Design review of the part built by this model. Coordinates are the model's own, in mm. A direction names the side the tool comes from. Round coordinates to 2 decimals unless told otherwise and drop trailing zeros. Loops run counter-clockwise (first coordinate to the right, second up) from the corner with the lowest first, then second, coordinate; pieces in that order, holes last. Notation, with made-up numbers: M 57,50.5 L 81,50.5 A18 ccw 81,79.5 Z; hole C 19.5,40.25 d10. An arc over 180 degrees is marked long. One line per item, written item: value. Start each with the question number.
Item 1: For line 1 along Y through (x, z) = (-13, -50); line 2 along X through (y, z) = (-44, 2); line 3 along X through (y, z) = (8.5, 7.5), list the stretches that pass through material, from the lowest coordinate up.
Item 2: We need section A-A (x = 30). Write out the cut boundary in (y, z), then the cut area to 3 significant figures.
Item 3: Mouldability with a two-part tool opening along X and no side actions: class faces 6 (the flat face through (-34, -39, 5)), 7 (the cylindrical face through (-15.542, -26.976, -49.909)), 8 (the cylindrical face through (-49, -26, -13)) as released by +X, released by -X, zero draft, split by the parting line, or undercut.
Item 4: We need section C-C (y = -44.5). Write out the cut boundary in (x, z).
Item 5: We need section D-D (z = -50.15). Write out the cut boundary in (x, y).
Item 6: Clearance check with flat-ended pins moving along their axes: pin 1 (12 mm diameter, centred on x = -17, z = -27, fed in from +Y); pin 2 (10 mm diameter, centred on x = 13, y = -21.5, fed in from -Z); pin 3 (2.5 mm diameter, centred on x = 29, y = -1, fed in from +Z). State where each tip first meets the part, or that it passes through.
Item 7: For faces 1 (the flat face through (-42.5, -33, 5)), 2 (the flat face through (-43, 4, 0)), 3 (the flat face through (-9, 7.84, -28)), 4 (the flat face through (-18.5, -20.13, -44.35)), 5 (the flat face through (-16, -36, -51.3)), list the 3-axis set-ups (+Z, -Z, +X, -X, +Y, -Y) from which the entire face can be reached by the end or side of a thin tool; tool diameter is ignored.
from build123d import *

# Parameters (mm, degrees)
SKETCH1_W            = 100
SKETCH1_H            = 60
SKETCH1_R            = 4.25
BOSS_EXTRUDE1_DEPTH  = 13.5
SKETCH2_R            = 7
BOSS_EXTRUDE2_DEPTH  = 10
CHAMFER1_SIZE        = 14
FILLET1_R            = 2.5
CUT_EXTRUDE1_DEPTH   = 12
SKETCH5_R            = 1.25
CUT_EXTRUDE2_DEPTH   = 12
SKETCH6_R            = 2.75
CUT_EXTRUDE3_DEPTH   = 10
CUT_EXTRUDE4_DEPTH   = 17
SKETCH11_W           = 17
SKETCH11_H           = 28.01
CUT_EXTRUDE5_DEPTH   = 28.0000001
SKETCH13_R           = 4.25
BOSS_EXTRUDE6_DEPTH  = 9
SKETCH14_R           = 1.85
SKETCH14_R_2         = 11.7
BOSS_EXTRUDE7_DEPTH  = 6
BOSS_EXTRUDE8_START  = 4
BOSS_EXTRUDE8_DEPTH  = 3
SKETCH17_W           = 6
SKETCH17_H           = 42.718705864
BOSS_EXTRUDE9_DEPTH  = 1
BOSS_EXTRUDE12_DEPTH = 3
SKETCH19_W           = 6
SKETCH19_H           = 24.5
BOSS_EXTRUDE13_DEPTH = 6
SKETCH21_W           = 6
SKETCH21_H           = 21.281155669
BOSS_EXTRUDE14_DEPTH = 3
BOSS_EXTRUDE15_DEPTH = 3
FILLET3_R            = 2


with BuildPart() as part:
    # Sketch1 → Boss-Extrude1 (new body, symmetric)
    with BuildSketch(Plane.XY):
        with Locations((0, -19)):
            Rectangle(SKETCH1_W, SKETCH1_H)
        with Locations((30, 0)):
            Circle(SKETCH1_R, mode=Mode.SUBTRACT)
        with Locations((-30, 0)):
            Circle(SKETCH1_R, mode=Mode.SUBTRACT)
    extrude(amount=BOSS_EXTRUDE1_DEPTH, both=True)

    # Sketch2 → Boss-Extrude2 (add)
    with BuildSketch(Plane(origin=(0, 0, -13.5), x_dir=(-1, 0, 0), z_dir=(0, 0, -1))):
        with Locations((-30, 0)):
            Circle(SKETCH2_R)
        with Locations((30, 0)):
            Circle(SKETCH2_R)
    extrude(amount=-BOSS_EXTRUDE2_DEPTH)

    # Chamfer1
    chamfer1_edges = [part.edges().sort_by_distance(p)[0] for p in [
        (-50, 11, 0),
        (50, 11, 0),
    ]]
    chamfer(chamfer1_edges, length=CHAMFER1_SIZE)

    # Fillet1
    fillet1_edges = [part.edges().sort_by_distance(p)[0] for p in [
        (-50, -26, -13.5),
        (-50, -26, 13.5),
        (0, 11, -13.5),
        (43, 4, -13.5),
        (-43, 4, -13.5),
        (0, 11, 13.5),
        (50, -26, 13.5),
        (43, 4, 13.5),
        (-43, 4, 13.5),
        (50, -26, -13.5),
    ]]
    fillet(fillet1_edges, radius=FILLET1_R)

    # Sketch3 → Cut-Extrude1 (cut)
    with BuildSketch(Plane.XY.offset(13.5)):
        Polygon((11.5, 1.5), (-11.5, 1.5), (-11.5, -14.75), (-11.5, -25.79), (11.5, -25.79), (11.5, -14.75), align=None)
    extrude(amount=-CUT_EXTRUDE1_DEPTH, mode=Mode.SUBTRACT)

    # Sketch5 → Cut-Extrude2 (cut)
    with BuildSketch(Plane(origin=(0, 11, 0), x_dir=(1, 0, 0), z_dir=(0, 1, 0))):
        with Locations((30, -7.5)):
            Circle(SKETCH5_R)
        with Locations((-30, -7.5)):
            Circle(SKETCH5_R)
    extrude(amount=-CUT_EXTRUDE2_DEPTH, mode=Mode.SUBTRACT)

    # Sketch6 → Cut-Extrude3 (cut)
    with BuildSketch(Plane.XZ.offset(49)):
        with Locations((36.277796695, 2.75)):
            Circle(SKETCH6_R)
    cut_extrude3 = extrude(amount=-CUT_EXTRUDE3_DEPTH, mode=Mode.SUBTRACT)

    # Sketch7 → Cut-Extrude4 (cut)
    with BuildSketch(Plane.XY.offset(13.5)):
        Polygon((42.5, -39), (30.5, -39), (25.5, -39), (25.5, -28), (30.5, -28), (42.5, -28), align=None)
    cut_extrude4 = extrude(amount=-CUT_EXTRUDE4_DEPTH, mode=Mode.SUBTRACT)

    # Mirror1: Cut-Extrude3, Cut-Extrude4 across plane
    add(cut_extrude3.mirror(Plane(origin=(0, 0, 0), x_dir=(0, 0, 1), z_dir=(1, 0, 0))), mode=Mode.SUBTRACT)
    add(cut_extrude4.mirror(Plane(origin=(0, 0, 0), x_dir=(0, 0, 1), z_dir=(1, 0, 0))), mode=Mode.SUBTRACT)

    # Sketch11 → Cut-Extrude5 (cut, through all)
    with BuildSketch(Plane(origin=(0, 0, -13.5), x_dir=(-1, 0, 0), z_dir=(0, 0, -1))):
        with Locations((0, -13.310174912)):
            Rectangle(SKETCH11_W, SKETCH11_H)
    extrude(amount=-CUT_EXTRUDE5_DEPTH, mode=Mode.SUBTRACT)

    # Sketch13 → Boss-Extrude6 (add)
    with BuildSketch(Plane.XY.offset(-3.5)):
        with Locations((30, 0)):
            Circle(SKETCH13_R)
        with Locations((-30, 0)):
            Circle(SKETCH13_R)
    extrude(amount=BOSS_EXTRUDE6_DEPTH)

    # Sketch14 → Boss-Extrude7 (add)
    with BuildSketch(Plane(origin=(-18.5, 0, 0), x_dir=(0, 0, -1), z_dir=(1, 0, 0))):
        Polygon((55.8, -29.960174912), (55.8, 3.339825088), (51.3, 7.839825088), (18, 7.839825088), (11, 7.839825088), (11, -34.460174912), (18, -34.460174912), (51.3, -34.460174912), align=None)
        with Locations((50.15, -28.810174912)):
            Circle(SKETCH14_R, mode=Mode.SUBTRACT)
        with Locations((50.15, 2.189825088)):
            Circle(SKETCH14_R, mode=Mode.SUBTRACT)
        with Locations((19.15, 2.189825088)):
            Circle(SKETCH14_R, mode=Mode.SUBTRACT)
        with Locations((19.15, -28.810174912)):
            Circle(SKETCH14_R, mode=Mode.SUBTRACT)
        with Locations((34.65, -13.310174912)):
            Circle(SKETCH14_R_2, mode=Mode.SUBTRACT)
    extrude(amount=BOSS_EXTRUDE7_DEPTH)

    # Sketch15 → Boss-Extrude8 (add)
    with BuildSketch(Plane.XZ.offset(34.460174912).offset(BOSS_EXTRUDE8_START)):
        Polygon((-14.5, -39.5), (20.060854185, -10.5), (-14.5, -10.5), align=None)
    extrude(amount=-BOSS_EXTRUDE8_DEPTH)

    # Sketch17 → Boss-Extrude9 (add)
    with BuildSketch(Plane.XZ.offset(34.460174912)):
        with Locations((-15.5, -29.940647068)):
            Rectangle(SKETCH17_W, SKETCH17_H)
    extrude(amount=BOSS_EXTRUDE9_DEPTH)

    # Sketch18 → Boss-Extrude12 (add)
    with BuildSketch(Plane.XZ.offset(35.460174912)):
        Polygon((-18.5, -10.5), (-41.575239857, -10.5), (-18.5, -38), (-13.739171521, -38), (-13.739171521, -10.5), align=None)
    extrude(amount=BOSS_EXTRUDE12_DEPTH)

    # Sketch19 → Boss-Extrude13 (add)
    with BuildSketch(Plane.XZ.offset(38.460174912)):
        with Locations((-15.5, -25.75)):
            Rectangle(SKETCH19_W, SKETCH19_H)
    extrude(amount=-BOSS_EXTRUDE13_DEPTH)

    # Sketch21 → Boss-Extrude14 (add)
    with BuildSketch(Plane.XZ.offset(35.460174912)):
        with Locations((-15.5, -40.659422166)):
            Rectangle(SKETCH21_W, SKETCH21_H)
    extrude(amount=BOSS_EXTRUDE14_DEPTH)

    # Sketch22 → Boss-Extrude15 (add)
    with BuildSketch(Plane(origin=(0, 7.839825088, 0), x_dir=(1, 0, 0), z_dir=(0, 1, 0))):
        Polygon((-12.5, 37.821800738), (-15.5, 37.821800738), (-15.5, 11), (-12.5, 11), (16.485593407, 11), (16.485593407, 13.5), align=None)
    extrude(amount=-BOSS_EXTRUDE15_DEPTH)

    # Fillet3
    fillet3_edges = [part.edges().sort_by_distance(p)[0] for p in [
        (-12.5, 6.339825088, -37.821800738),
        (-39.057940964, -36.960174912, -13.5),
        (-18.5, -36.960174912, -38),
        (16.485593407, 6.339825088, -13.5),
        (16.485593407, -36.960174912, -13.5),
        (-12.5, -36.960174912, -37.821800738),
        (-11.286173778, -38.460174912, -13.5),
        (-12.5, -35.460174912, -25.660900369),
        (1.992796704, -35.460174912, -13.5),
        (-12.5, -15.310174912, -13.5),
        (1.992796704, 4.839825088, -13.5),
    ]]
    fillet(fillet3_edges, radius=FILLET3_R)


solid = part.part
A:
1. line 1: -38.46 to -30.65, -26.97 to 0.35, 4.03 to 7.84
1. line 2: -50 to -38.92, -33.63 to 33.63, 38.92 to 50
1. line 3: -38.5 to -31.25, -28.75 to 28.75, 31.25 to 38.5
2. outline: M -49,-13.5 L 8.5,-13.5 A2.5 ccw 11,-11 L 11,6.25 L 4.25,6.25 L 4.25,5.5 L -4.25,5.5 L -4.25,13.5 L -28,13.5 L -28,-3.5 L -39,-3.5 L -39,13.5 L -49,13.5 Z; M 4.25,8.75 L 11,8.75 L 11,11 A2.5 ccw 8.5,13.5 L 4.25,13.5 Z
2. area: 1,350 mm2
3. face 6: undercut
3. face 7: zero draft
3. face 8: released by -X
4. outline: M -50,-11 A2.5 ccw -47.5,-13.5 L 47.5,-13.5 A2.5 ccw 50,-11 L 50,11 A2.5 ccw 47.5,13.5 L -47.5,13.5 A2.5 ccw -50,11 Z; hole C -36.28,2.75 d5.5; hole C 36.28,2.75 d5.5
5. outline: M -18.5,-38.46 L -12.5,-38.46 L -12.5,-30.66 L -18.5,-30.66 Z; M -18.5,-26.96 L -12.5,-26.96 L -12.5,0.34 L -18.5,0.34 Z; M -18.5,4.04 L -12.5,4.04 L -12.5,7.84 L -18.5,7.84 Z
6. pin 1: y = 7.84
6. pin 2: z = -13.5
6. pin 3: z = 5.5
7. face 1: +Z
7. face 2: +Z, -Z, -X, +Y
7. face 3: -Z, +X, -X, +Y
7. face 4: -Z, -X, +Y
7. face 5: -Z, +X, -X, -Y
